Can you work these out from the model? Positions are in its coordinate system, mm. Round coordinates to 2 decimals unless told otherwise and drop trailing zeros. Write each loop counter-clockwise with the first axis right and the second up, starting at its lowest first coordinate (ties: lowest second). Pieces come first, ordered by that corner, then holes. Notation, with made-up numbers: M 18,57 L 41,57 A4 cw 41,62 Z; hole C 34.25,20.25 d11. An arc over 180 degrees is marked long. Use one line per item in the form item = value. Start each with the question number.
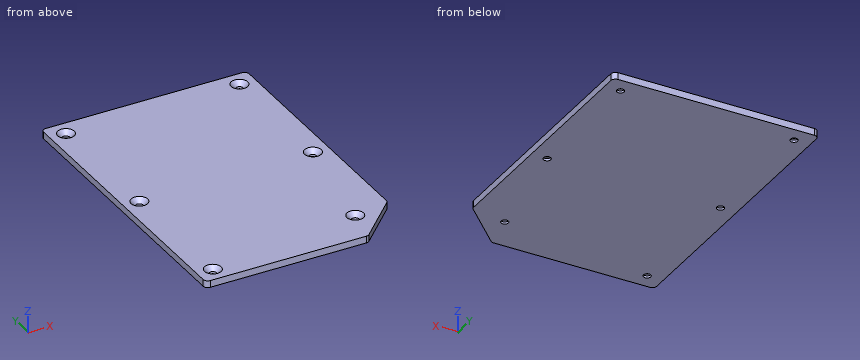
```python
from build123d import *

# Parameters (mm, degrees)
BOSS_EXTRUDE1_DEPTH                                 = 3
CSK_FOR_M3_COUNTERSUNK_FLAT_HEAD_SCREW1_D           = 3.2
CSK_FOR_M3_COUNTERSUNK_FLAT_HEAD_SCREW1_DEPTH       = 5
CSK_FOR_M3_COUNTERSUNK_FLAT_HEAD_SCREW1_CSINK_D     = 7.3
CSK_FOR_M3_COUNTERSUNK_FLAT_HEAD_SCREW1_CSINK_ANGLE = 90
CSK_FOR_M3_COUNTERSUNK_FLAT_HEAD_SCREW1_TIP         = 0.96137699


with BuildPart() as part:
    # Sketch1 → Boss-Extrude1 (new body)
    with BuildSketch(Plane.XY):
        with BuildLine():
            Line((-43, 70), (43, 70))
            ThreePointArc((43, 70), (44.414213562, 69.414213562), (45, 68))
            Line((45, 68), (45, -40.384776311))
            ThreePointArc((45, -40.384776311), (44.847759065, -41.150143176), (44.414213562, -41.798989873))
            Line((44.414213562, -41.798989873), (26.798989873, -59.414213562))
            ThreePointArc((26.798989873, -59.414213562), (26.150143176, -59.847759065), (25.384776311, -60))
            Line((25.384776311, -60), (-43, -60))
            ThreePointArc((-43, -60), (-44.414213562, -59.414213562), (-45, -58))
            Line((-45, -58), (-45, 68))
            ThreePointArc((-45, 68), (-44.414213562, 69.414213562), (-43, 70))
        make_face()
    extrude(amount=BOSS_EXTRUDE1_DEPTH)

    # CSK for M3 Countersunk Flat Head Screw1
    with Locations(Plane(origin=(-38, -53, 3), x_dir=(1, 0, 0), z_dir=(0, 0, 1))):
        with Locations((0, 0), (67.242640687, 8.757359313), (76, 58), (0, 58), (0, 116), (76, 116)):
            CounterSinkHole(CSK_FOR_M3_COUNTERSUNK_FLAT_HEAD_SCREW1_D / 2, CSK_FOR_M3_COUNTERSUNK_FLAT_HEAD_SCREW1_CSINK_D / 2, depth=CSK_FOR_M3_COUNTERSUNK_FLAT_HEAD_SCREW1_DEPTH, counter_sink_angle=CSK_FOR_M3_COUNTERSUNK_FLAT_HEAD_SCREW1_CSINK_ANGLE)
            with Locations((0, 0, -(CSK_FOR_M3_COUNTERSUNK_FLAT_HEAD_SCREW1_DEPTH + CSK_FOR_M3_COUNTERSUNK_FLAT_HEAD_SCREW1_TIP / 2))):  # 118° drill point
                Cone(0, CSK_FOR_M3_COUNTERSUNK_FLAT_HEAD_SCREW1_D / 2, CSK_FOR_M3_COUNTERSUNK_FLAT_HEAD_SCREW1_TIP, mode=Mode.SUBTRACT)


solid = part.part
```
1. If we section it at C-C (x = 38): List the corners of the cut face in (y, z) for me, and give its area (3 significant figures).
2. Please list where these lines run through material, in increasing order: line 1 along X through (y, z) = (63, 0.4); line 2 along Y through (x, z) = (-38, 0.2); line 3 along Y through (x, z) = (-39, 1.05).
3. If we section it at A-A (x = -38): List the corners of the cut face in (y, z) for me, and give its area (3 significant figures).
4. If we section it at B-B (z = 2.3): List the corners of the cut face in (x, y) for me.
5. Will these pins go through, and if not, where does the flat tip stop? pin 1 (1.5 mm diameter, centred on x = 32.5, z = 1, fed in from -Y); pin 2 (4 mm diameter, centred on x = 38, y = 63, fed in from +Z).
Model answer:
q1.outline = M -48.21,0 L 3.4,0 L 3.4,0.95 L 1.35,3 L -48.21,3 Z; M 6.6,0 L 61.4,0 L 61.4,0.95 L 59.35,3 L 8.65,3 L 6.6,0.95 Z; M 64.6,0 L 70,0 L 70,3 L 66.65,3 L 64.6,0.95 Z
q1.area = 327 mm2
q2.line_1 = -45 to -39.6, -36.4 to 36.4, 39.6 to 45
q2.line_2 = -60 to -54.6, -51.4 to 3.4, 6.6 to 61.4, 64.6 to 70
q2.line_3 = -60 to -54.37, -51.63 to 3.63, 6.37 to 61.63, 64.37 to 70
q3.outline = M -60,0 L -54.6,0 L -54.6,0.95 L -56.65,3 L -60,3 Z; M -51.4,0 L 3.4,0 L 3.4,0.95 L 1.35,3 L -49.35,3 L -51.4,0.95 Z; M 6.6,0 L 61.4,0 L 61.4,0.95 L 59.35,3 L 8.65,3 L 6.6,0.95 Z; M 64.6,0 L 70,0 L 70,3 L 66.65,3 L 64.6,0.95 Z
q3.area = 349 mm2
q4.outline = M -45,-58 A2 ccw -43,-60 L 25.38,-60 A2 ccw 26.8,-59.41 L 44.41,-41.8 A2 ccw 45,-40.38 L 45,68 A2 ccw 43,70 L -43,70 A2 ccw -45,68 Z; hole C -38,-53 d5.9; hole C -38,5 d5.9; hole C -38,63 d5.9; hole C 29.24,-44.24 d5.9; hole C 38,5 d5.9; hole C 38,63 d5.9
q5.pin_1 = -54.46
q5.pin_2 = 1.35
